Autodesk Inventor part; units mm, degrees
ref_plane "YZ Plane" through (0, 0, 0) normal (1, 0, 0) x (0, 1, 0)
ref_plane "XZ Plane" through (0, 0, 0) normal (0, 1, 0) x (-1, 0, 0)
ref_plane "XY Plane" through (0, 0, 0) normal (0, 0, 1) x (1, 0, 0)
sketch "スケッチ1" plane through (0, 0, 0) normal (0, 1, 0) x (-1, 0, 0)
  line L0 (0, 0) -> (-154, 0)
  line L1 (-154, 0) -> (-154, 178.952)
  line L2 (-154, 178.952) -> (0, 178.952)
  line L3 (0, 178.952) -> (0, 0)
  dimension "d0" = 178.952
  dimension "d1" = 154
extrude "押し出し1" add sketch "スケッチ1" along normal blind 3
sketch "スケッチ2" plane through (0, 3, 0) normal (0, 1, 0) x (1, 0, 0)
  line L0 (0, 0) -> (0, -178.952)
  line L1 (0, -163.952) -> (154, -163.952)
  line L2 (154, -178.952) -> (154, 0)
  line L3 (0, -178.952) -> (154, -178.952)
  line L4 (0, -118.952) -> (154, -118.952)
  line L5 (0, -15) -> (154, -15)
  line L6 (154, 0) -> (0, 0)
  line L7 (0, -60) -> (154, -60)
  line L8 (5, -178.952) -> (5, 0)
  line L9 (149, -178.952) -> (149, -168.1662)
  line L10 (149, -168.1662) -> (149, 0)
  point P0 (5, -163.952)
  point P1 (5, -118.952)
  point P2 (5, -60)
  point P3 (5, -15)
  point P4 (149, -15)
  point P5 (149, -60)
  point P6 (149, -118.952)
  point P7 (149, -163.952)
  dimension "d4" = 15
  dimension "d5" = 45
  dimension "d6" = 15
  dimension "d7" = 45
  dimension "d8" = 5
  dimension "d9" = 5
hole "穴1" at (5, 3, 163.952) at (5, 3, 118.952) at (5, 3, 60) at (5, 3, 15) at (149, 3, 15) at (149, 3, 60) at (149, 3, 118.952) at (149, 3, 163.952) direction (0, -1, 0) diameter 3.1 end through all
sketch "スケッチ3" plane through (0, 3, 0) normal (0, 1, 0) x (1, 0, 0)
  circle A0 centre (5, -118.952) radius 1.55
  circle A1 centre (149, -118.952) radius 1.55
  line L0 (5, -118.952) -> (149, -118.952)
  circle A2 centre (149, -60) radius 1.55
  line L1 (149, -118.952) -> (149, -60)
  circle A3 centre (5, -60) radius 1.55
  line L2 (149, -60) -> (5, -60)
  line L3 (5, -60) -> (5, -118.952)
  line L4 (5, -90.476) -> (149, -90.476)
  line L5 (77, -118.952) -> (77, -60)
  circle A4 centre (77, -90.476) radius 15.18
  line L6 (5, -89.476) -> (149, -89.476)
  point P0 (0, 0)
  point P1 (61.82, -90.476)
  point P2 (63.8537, -98.066)
  point P3 (69.41, -103.6223)
  point P4 (77, -105.656)
  point P5 (84.59, -103.6223)
  point P6 (90.1463, -98.066)
  point P7 (92.18, -90.476)
  point P8 (90.1463, -82.886)
  point P9 (84.59, -77.3297)
  point P10 (77, -75.296)
  point P11 (69.41, -77.3297)
  point P12 (63.8537, -82.886)
  dimension "d18" = 30.36
  dimension "d21" = 360
  dimension "d50" = 1
hole "穴2" at (61.82, 3, 90.476) at (63.8537, 3, 98.066) at (69.41, 3, 103.6223) at (77, 3, 105.656) at (84.59, 3, 103.6223) at (90.1463, 3, 98.066) at (92.18, 3, 90.476) at (90.1463, 3, 82.886) at (84.59, 3, 77.3297) at (77, 3, 75.296) at (69.41, 3, 77.3297) at (63.8537, 3, 82.886) direction (0, -1, 0) diameter 4.1 end through all
sketch "スケッチ4" plane through (0, 3, 0) normal (0, 1, 0) x (1, 0, 0)
  circle A0 centre (77, -75.296) radius 2.05
  circle A1 centre (77, -105.656) radius 2.05
  line L0 (77, -75.296) -> (77, -105.656)
  circle A2 centre (77, -90.476) radius 9
  point P0 (0, 0)
  dimension "d30" = 18
extrude "押し出し2" cut sketch "スケッチ4" against normal blind 3 contours A2 L0 | L0 A2
sketch "スケッチ5" plane through (0, 3, 0) normal (0, 1, 0) x (1, 0, 0)
  circle A0 centre (77, -90.476) radius 9
  circle A1 centre (77, -90.476) radius 88
  line L0 (77, -90.476) -> (77, -178.476)
  line L1 (77, -90.476) -> (14.7746, -152.7014)
  point P0 (0, 0)
  point P1 (139.2254, -152.7014)
  point P2 (139.2254, -28.2506)
  point P3 (14.7746, -28.2506)
  dimension "d36" = 176
  dimension "d37" = 45
  dimension "d40" = 360
hole "穴3" at (14.7746, 3, 152.7014) at (139.2254, 3, 152.7014) at (139.2254, 3, 28.2506) at (14.7746, 3, 28.2506) direction (0, -1, 0) diameter 4.1 end through all
sketch "スケッチ6" plane through (0, 3, 0) normal (0, 1, 0) x (1, 0, 0)
  line L0 (0, -178.952) -> (154, -178.952)
  line L1 (144, -178.952) -> (144, 0)
  line L2 (154, 0) -> (0, 0)
  line L3 (154, -178.952) -> (154, 0)
  line L4 (10, -178.952) -> (10, 0)
  line L5 (0, 0) -> (0, -178.952)
  circle A0 centre (77, -90.476) radius 9
  circle A1 centre (77, -90.476) radius 25
  line L6 (129, -163.952) -> (25, -163.952)
  line L7 (25, -163.952) -> (25, -15)
  line L8 (25, -15) -> (129, -15)
  line L9 (129, -15) -> (129, -163.952)
  line L10 (77, -90.476) -> (25, -163.952)
  line L11 (77, -90.476) -> (129, -15)
  line L12 (77, -90.476) -> (25, -15)
  line L13 (77, -90.476) -> (129, -163.952)
  line L14 (129, -150.969) -> (96.8988, -105.61)
  line L15 (119.8118, -163.952) -> (84.6548, -114.2752)
  line L16 (96.7064, -75.0923) -> (129, -28.2195)
  line L17 (84.3542, -66.5822) -> (119.8923, -15)
  line L18 (69.6458, -66.5822) -> (34.1077, -15)
  line L19 (57.2936, -75.0923) -> (25, -28.2195)
  line L20 (69.3452, -114.2752) -> (34.1882, -163.952)
  line L21 (57.1012, -105.61) -> (25, -150.969)
  line L22 (53.1515, -97.976) -> (25, -97.976)
  line L23 (53.1515, -82.976) -> (25, -82.976)
  line L24 (77, -90.476) -> (10, -90.476)
  line L25 (77, -90.476) -> (77, -163.952)
  line L26 (100.8485, -97.976) -> (129, -97.976)
  line L27 (100.8485, -82.976) -> (129, -82.976)
  point P0 (100.8485, -97.976)
  dimension "d53" = 50
  dimension "d51" = 10
  dimension "d52" = 10
  dimension "d54" = 15
  dimension "d55" = 15
  dimension "d56" = 15
  dimension "d57" = 15
  dimension "d58" = 7.5
  dimension "d59" = 7.5
  dimension "d60" = 7.5
  dimension "d61" = 7.5
  dimension "d62" = 7.5
  dimension "d63" = 7.5
  dimension "d64" = 7.5
  dimension "d65" = 7.5
  dimension "d69" = 7.5
  dimension "d70" = 7.5
extrude "押し出し3" cut sketch "スケッチ6" against normal blind 3 contours L22 A1 L21 L7 | L7 L19 A1 L23 | L20 A1 L25 L6 | L8 L17 A1 L18 | L25 A1 L15 L6 | L16 L9 L27 A1 | A1 L26 L9 L14
fillet "フィレット1" radius 10 4 edges at (0, 1.5, 0) (0, 1.5, 178.952) (154, 1.5, 178.952) (154, 1.5, 0)
properties part number "base_plate5" material "アルミニウム 6061"
Could you check a few things on this model? Use its own coordinates, in mm. A direction names the side the tool comes from. Round coordinates to 2 decimals unless told otherwise and drop trailing zeros. Loops run counter-clockwise (first coordinate to the right, second up) from the corner with the lowest first, then second, coordinate; pieces in that order, holes last.
Q1. Thinking about a two-plate mould opening in X: for faces 1 (the flat face through (102.48, 1.52, 139.46)), 2 (the cylindrical face through (3.01, 1.52, 2.85)), which applies, pulls with the +X half, pulls with the -X half, needs draft (parallel to the pull), parting line crosses it, or undercut?
Q2. I want a section at A-A (x = 77). Write out the boundary of the cut face in (y, z), and give its area (3 significant figures).
Q3. I want a section at B-B (z = 135). Write out the boundary of the cut face in (x, y).
Q4. I want a section at C-C (x = 30.5). Write out the boundary of the cut face in (y, z), and give its area (3 significant figures).
Q5. On a 3-axis mill with a long thin cutter (end or side, diameter ignored), from which of +Z, -Z, +X, -X, +Y, -Y can I reach the whole of each face in a straight line? I mean faces 3 (the flat face through (41.37, 1.52, 51.98)), 4 (the cylindrical face through (2.852, 1.521, 175.945)). Say none if no direction works.
Q6. I want a section at D-D (x = 47). Write out the boundary of the cut face in (y, z), and give its area (3 significant figures).
Q7. Please list where these lines run through material, in increasing order: L1, parallel to Z at x = 89.5, y = 0.5; L2, parallel to X at y = 1.8, z = 51.5; L3, parallel to Z at x = 56.5, y = 1.
Answer below:
1. face 1: undercut
1. face 2: pulls with the -X half
2. outline: (0, 0) - (3, 0) - (3, 15) - (0, 15) - close; (0, 65.48) - (3, 65.48) - (3, 73.25) - (0, 73.25) - close; (0, 77.35) - (3, 77.35) - (3, 81.48) - (0, 81.48) - close; (0, 99.48) - (3, 99.48) - (3, 103.61) - (0, 103.61) - close; (0, 107.71) - (3, 107.71) - (3, 115.48) - (0, 115.48) - close; (0, 163.95) - (3, 163.95) - (3, 178.95) - (0, 178.95) - close
2. area: 161 mm2
3. outline: (0, 0) - (25, 0) - (25, 3) - (0, 3) - close; (36.3, 0) - (54.68, 0) - (54.68, 3) - (36.3, 3) - close; (99.32, 0) - (117.7, 0) - (117.7, 3) - (99.32, 3) - close; (129, 0) - (154, 0) - (154, 3) - (129, 3) - close
4. outline: (0, 0) - (3, 0) - (3, 36.2) - (0, 36.2) - close; (0, 82.98) - (3, 82.98) - (3, 97.98) - (0, 97.98) - close; (0, 143.2) - (3, 143.2) - (3, 178.95) - (0, 178.95) - close
4. area: 261 mm2
5. face 3: +Y, -Y
5. face 4: +Z, -X, +Y, -Y
6. outline: (0, 0) - (3, 0) - (3, 15) - (0, 15) - close; (0, 33.71) - (3, 33.71) - (3, 60.15) - (0, 60.15) - close; (0, 82.98) - (3, 82.98) - (3, 97.98) - (0, 97.98) - close; (0, 119.88) - (3, 119.88) - (3, 145.85) - (0, 145.85) - close; (0, 163.95) - (3, 163.95) - (3, 178.95) - (0, 178.95) - close
6. area: 292 mm2
7. L1: z = 0 to 15, 59.11 to 80.94, 84.83 to 96.12, 100.01 to 121.12, 163.95 to 178.95
7. L2: x = 0 to 25, 41.04 to 59.25, 94.75 to 112.96, 129 to 154
7. L3: z = 0 to 15, 47.5 to 73.94, 76.17 to 104.79, 106.46 to 132.43, 163.95 to 178.95
